The figure shows three views and two pictorial views of one solid part (mm, origin at its lowest corner). Answer the questions. Round coordinates to 2 decimals unless told otherwise and drop trailing zeros. Order: outer loops, then holes, each group sorted by start corner. A loop starts at its lowest first (then second) coordinate and runs counter-clockwise, first axis right, second up. Notation, with made-up numbers: (74, -25.75) -> (86, -25.75) arc R35 ccw to (86, 7.25) -> close; hole circle Ø5 at (20.5, -38). An arc over 180 degrees is marked (long way). One line per item, written item: value. Start each with the question number.
1. The mould has two halves that part along Y. Classify the marked faces 1, 2, 3 and 4: released by +Y, released by -Y, zero draft, split by the parting line, or undercut.
2. Consider line 1 (X direction, y = 0.75, z = 19.5); line 2 (Z direction, x = 58.5, y = 2); line 3 (Y direction, x = 18, z = 98). Determine where each line is inside the solid, lowest interval first.
3. Section A-A (x = 43) is taken. Give the vertices of the cut face in (y, z).
4. Section C-C (y = 5) is taken. Give the vertices of the cut face in (x, z).
5. Section B-B (z = 44) is taken. Give the vertices of the cut face in (x, y), then the cut area to 3 significant figures.
6. Flat-ended cylindrical pins translate along their axes: pin 1 Ø1.5 at (x, y) = (53.5, 11) entering from -Z; pin 2 Ø3 at (x, z) = (19, 95.5) entering from +Y; pin 3 Ø3.5 at (y, z) = (7.5, 36.5) entering from -X. Find the tip coordinate at first contact, or state that the pin passes through.
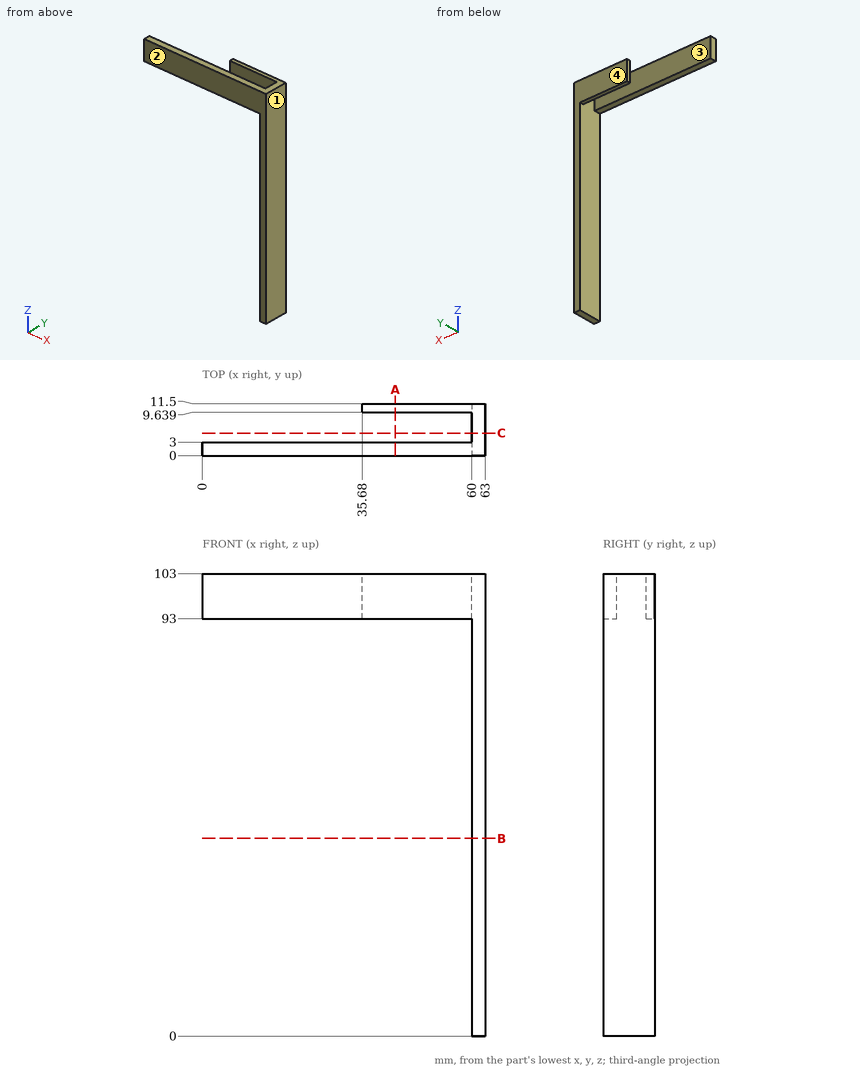
Answer:
1. face 1: zero draft
1. face 2: released by -Y
1. face 3: undercut
1. face 4: released by +Y
2. line 1: 60 to 63
2. line 2: 93 to 103
2. line 3: 0 to 3
3. outline: (0, 93) -> (3, 93) -> (3, 103) -> (0, 103) -> close; (9.64, 93) -> (11.5, 93) -> (11.5, 103) -> (9.64, 103) -> close
4. outline: (60, 0) -> (63, 0) -> (63, 103) -> (60, 103) -> close
5. outline: (60, 0) -> (63, 0) -> (63, 11.5) -> (60, 11.5) -> close
5. area: 34.5 mm^2
6. pin 1: z = 93
6. pin 2: y = 3
6. pin 3: x = 60
